CAD build for the part. Positions are in the model's coordinates, mm. A direction names the side the tool comes from. Coordinates: 2 decimals unless noted, no trailing zeros. Order: outer loops, then holes, each group sorted by start corner. A loop starts at its lowest first (then second) coordinate and runs counter-clockwise, first axis right, second up. Notation, with made-up numbers: M 62,3.25 L 90,3.25 A7 ccw 90,10.25 Z; hole C 30.25,23 d2. An arc over 180 degrees is marked long. Write item = value, one per line.
from build123d import *

# Parameters (mm, degrees)
BOSS_EXTRUDE4_DEPTH = 5
SKETCH6_W           = 70
SKETCH6_H           = 70
BOSS_EXTRUDE5_DEPTH = 30
SKETCH8_R           = 3
CUT_EXTRUDE1_DEPTH  = 2
CUT_EXTRUDE3_START  = -30
CUT_EXTRUDE3_DEPTH  = 30
SKETCH10_W          = 140
SKETCH10_H          = 140
BOSS_EXTRUDE6_DEPTH = 2.5
FILLET1_R           = 10
CHAMFER1_SIZE       = 1.25


with BuildPart() as part:
    # Sketch5 → Boss-Extrude4 (new body)
    with BuildSketch(Plane(origin=(0, 0, 0), x_dir=(1, 0, 0), z_dir=(0, 1, 0))):
        with BuildLine():
            Line((-22.5, -32.5), (22.5, -32.5))
            ThreePointArc((22.5, -32.5), (29.571067812, -29.571067812), (32.5, -22.5))
            Line((32.5, -22.5), (32.5, 22.5))
            ThreePointArc((32.5, 22.5), (29.571067812, 29.571067812), (22.5, 32.5))
            Line((22.5, 32.5), (-22.5, 32.5))
            ThreePointArc((-22.5, 32.5), (-29.571067812, 29.571067812), (-32.5, 22.5))
            Line((-32.5, 22.5), (-32.5, -22.5))
            ThreePointArc((-32.5, -22.5), (-29.571067812, -29.571067812), (-22.5, -32.5))
        make_face()
    extrude(amount=BOSS_EXTRUDE4_DEPTH)

    # Sketch6 → Boss-Extrude5 (add)
    with BuildSketch(Plane(origin=(0, 5, 0), x_dir=(1, 0, 0), z_dir=(0, 1, 0))):
        Rectangle(SKETCH6_W, SKETCH6_H)
    extrude(amount=BOSS_EXTRUDE5_DEPTH)

    # Sketch8 → Cut-Extrude1 (cut)
    with BuildSketch(Plane.XZ):
        with Locations(Location((26.037533906, -26.035533906, 0), (0, 0, 270))):
            Circle(SKETCH8_R)
        with Locations(Location((26.036533906, 26.036533906, 0), (0, 0, 270))):
            Circle(SKETCH8_R)
        with BuildLine():
            ThreePointArc((-23.035533906, 26.035533906), (-24.887483609, 28.807172503), (-28.156854249, 28.156854249))
            Line((-28.156854249, 28.156854249), (-23.914213562, 23.914213562))
            ThreePointArc((-23.914213562, 23.914213562), (-23.263895308, 24.887483609), (-23.035533906, 26.035533906))
        make_face()
        with BuildLine():
            Line((-23.914213562, 23.914213562), (-28.156854249, 28.156854249))
            ThreePointArc((-28.156854249, 28.156854249), (-28.156854249, 23.914213562), (-23.914213562, 23.914213562))
        make_face()
        with Locations(Location((-26.034533906, -26.036533906, 0), (0, 0, 270))):
            Circle(SKETCH8_R)
    extrude(amount=-CUT_EXTRUDE1_DEPTH, mode=Mode.SUBTRACT)

    # Mirror1: part across plane


with BuildPart() as part_1:
    add(part.part)
    add(part.part.mirror(Plane(origin=(-35, 35, -35), x_dir=(0, 0, 1), z_dir=(1, 0, 0))))

    # Mirror2: part across plane


with BuildPart() as part_2:
    add(part_1.part)
    add(part_1.part.mirror(Plane(origin=(35, 35, 35), x_dir=(1, 0, 0), z_dir=(0, 0, -1))))

    # Sketch9 → Cut-Extrude3 (cut)
    with BuildSketch(Plane(origin=(0, 35, 0), x_dir=(1, 0, 0), z_dir=(0, 1, 0)).offset(CUT_EXTRUDE3_START)):
        with BuildLine():
            Line((22.5, 32.5), (-92.5, 32.5))
            ThreePointArc((-92.5, 32.5), (-99.571067812, 29.571067812), (-102.5, 22.5))
            Line((-102.5, 22.5), (-102.5, -92.5))
            ThreePointArc((-102.5, -92.5), (-99.571067812, -99.571067812), (-92.5, -102.5))
            Line((-92.5, -102.5), (22.5, -102.5))
            ThreePointArc((22.5, -102.5), (29.571067812, -99.571067812), (32.5, -92.5))
            Line((32.5, -92.5), (32.5, 22.5))
            ThreePointArc((32.5, 22.5), (29.571067812, 29.571067812), (22.5, 32.5))
        make_face()
    extrude(amount=CUT_EXTRUDE3_DEPTH, mode=Mode.SUBTRACT)


with BuildPart() as cut_extrude3_piece_1:
    # of the separate pieces the step leaves, piece 1, a body of its own (cut_extrude3_pieces)
    add(part_2.part.solids().sort_by_distance((35, 5, -35))[0])

    # Sketch10 → Boss-Extrude6 (add)
    with BuildSketch(Plane.XZ.offset(-5)):
        with Locations((-35, 35)):
            Rectangle(SKETCH10_W, SKETCH10_H)
    extrude(amount=-BOSS_EXTRUDE6_DEPTH)


with BuildPart() as cut_extrude3_piece_2:
    # of the separate pieces the step leaves, piece 2, a body of its own (cut_extrude3_pieces)
    add(part_2.part.solids().sort_by_distance((32.5, 0, 22.5))[0])


with BuildPart() as cut_extrude3_piece_3:
    # of the separate pieces the step leaves, piece 3, a body of its own (cut_extrude3_pieces)
    add(part_2.part.solids().sort_by_distance((-92.5, 0, -32.5))[0])


with BuildPart() as cut_extrude3_piece_4:
    # of the separate pieces the step leaves, piece 4, a body of its own (cut_extrude3_pieces)
    add(part_2.part.solids().sort_by_distance((-102.5, 0, 47.5))[0])


with BuildPart() as cut_extrude3_piece_5:
    # of the separate pieces the step leaves, piece 5, a body of its own (cut_extrude3_pieces)
    add(part_2.part.solids().sort_by_distance((22.5, 0, 102.5))[0])


with BuildPart() as cut_extrude3_piece_4_1:
    add(cut_extrude3_piece_4.part)

    # Combine1: union Cut-Extrude3 piece 2, Cut-Extrude3 piece 3, Cut-Extrude3 piece 5, Cut-Extrude3 piece 1
    add(cut_extrude3_piece_2.part)
    add(cut_extrude3_piece_3.part)
    add(cut_extrude3_piece_5.part)
    add(cut_extrude3_piece_1.part)

    # Fillet1
    fillet1_edges = [cut_extrude3_piece_4_1.edges().sort_by_distance(p)[0] for p in [
        (35, 20, -35),
        (-105, 20, -35),
        (-105, 20, 105),
        (35, 20, 105),
    ]]
    fillet(fillet1_edges, radius=FILLET1_R)

    # Chamfer1
    chamfer1_edges = [cut_extrude3_piece_4_1.edges().sort_by_distance(p)[0] for p in [
        (-35, 35, 102.5),
        (-99.571067812, 35, 99.571067812),
        (-102.5, 35, 35),
        (29.571067812, 35, 99.571067812),
        (32.5, 35, 35),
        (-35, 35, -32.5),
        (-99.571067812, 35, -29.571067812),
        (29.571067812, 35, -29.571067812),
        (-102.5, 7.5, 35),
        (-99.571067812, 7.5, 99.571067812),
        (-35, 7.5, 102.5),
        (29.571067812, 7.5, 99.571067812),
        (32.5, 7.5, 35),
        (29.571067812, 7.5, -29.571067812),
        (-35, 7.5, -32.5),
        (-99.571067812, 7.5, -29.571067812),
    ]]
    chamfer(chamfer1_edges, length=CHAMFER1_SIZE)


solid = cut_extrude3_piece_4_1.part
(1) Slice it at D-D, the plane z = 34.5. Write the cut outline in (x, y), then the cut area to 4 significant figures.
Evaluation:
outline = M -105,5 L 35,5 L 35,35 L 33.75,35 L 32.5,33.75 L 32.5,8.75 L 31.25,7.5 L -101.25,7.5 L -102.5,8.75 L -102.5,33.75 L -103.75,35 L -105,35 Z
area = 487.5 mm²
(2) Slice it at A-A, the plane y = 14.5. Write the cut outline in (x, z), then the cut area to 4 significant figures.
Evaluation:
outline = M -105,-25 A10 ccw -95,-35 L 25,-35 A10 ccw 35,-25 L 35,95 A10 ccw 25,105 L -95,105 A10 ccw -105,95 Z; hole M -102.5,-22.5 A10 ccw -92.5,-32.5 L 22.5,-32.5 A10 ccw 32.5,-22.5 L 32.5,92.5 A10 ccw 22.5,102.5 L -92.5,102.5 A10 ccw -102.5,92.5 Z
area = 1,375 mm²
(3) Tool access for faces 1 (the face through (-102.5, 2, 0)), 2 (the face through (-96, 2, 44)), 3 (the face through (32.5, 21, 36)), 4 (the face through (0, 2, 32.5)), 5 (the face through (32.5, 2, 0)): list every direction of +Z, -Z, +X, -X, +Y, -Y with a clear straight run to the whole face (end or side of a thin tool).
Evaluation:
face_1 = +Z, -Z, -X, -Y
face_2 = -Y
face_3 = +Y
face_4 = +X, -X, -Y
face_5 = +Z, -Z, +X, -Y
(4) Slice it at C-C, the plane x = -62. Write the cut outline in (y, z), then the cut area to 3 significant figures.
Evaluation:
outline = M 0,-32.5 L 5,-32.5 L 5,-35 L 35,-35 L 35,-33.75 L 33.75,-32.5 L 8.75,-32.5 L 7.5,-31.25 L 7.5,101.25 L 8.75,102.5 L 33.75,102.5 L 35,103.75 L 35,105 L 5,105 L 5,102.5 L 0,102.5 L 0,37.5 L 5,37.5 L 5,32.5 L 0,32.5 Z
area = 1,140 mm²
(5) Wall check: line 1 (Z direction, x = -58.5, y = 27); line 2 (X direction, y = 22, z = 24); line 3 (Y direction, x = -4, z = 53). Give the ranges that are in metal, low to high. Write a range as from..to.
Evaluation:
line_1 = -35..-32.5, 102.5..105
line_2 = -105..-102.5, 32.5..35
line_3 = 0..7.5
(6) Slice it at B-B, the plane z = 7. Write the cut outline in (x, y).
Evaluation:
outline = M -105,5 L -102.5,5 L -102.5,0 L -37.5,0 L -37.5,5 L -32.5,5 L -32.5,0 L 32.5,0 L 32.5,5 L 35,5 L 35,35 L 33.75,35 L 32.5,33.75 L 32.5,8.75 L 31.25,7.5 L -101.25,7.5 L -102.5,8.75 L -102.5,33.75 L -103.75,35 L -105,35 Z
(7) Pin check, flat tips, straight feed: pin 1 Ø7 at (x, z) = (26.04, 43.96) entering from +Y; pin 2 Ø3 at (x, z) = (27, 95.5) entering from -Y; pin 3 Ø1.5 at (x, y) = (-30, 3.5) entering from -Z. Stop position of each tip, or through.
Evaluation:
pin_1 = 7.5
pin_2 = 2
pin_3 = -29.88
(8) Pull direction X, two halves, no side cores. Call faces 6 (the face through (24.212, 0.986, -23.655)), 7 (the face through (-34, 20, -35)), 8 (the face through (-98.76, 7.7, 98.9)), 9 (the face through (-102.5, 2, 70)): +X half, -X half, draft (parallel to the pull), parting line (faces both ways), or undercut.
Evaluation:
face_6 = undercut
face_7 = draft
face_8 = undercut
face_9 = -X half
